For this review, take the finished solid that the model builds, in its own axes (mm). Face numbers are marked on the shaded views. A direction names the side the tool comes from. Round coordinates to 2 decimals unless told otherwise and drop trailing zeros. Write each loop counter-clockwise with the first axis right and the second up, starting at its lowest first coordinate (ties: lowest second). Pieces come first, ordered by that corner, then holes. Notation, with made-up numbers: (29, -37) -> (65, -37) arc R12 ccw to (65, -29) -> close; hole circle Ø9 at (14.5, 20). An arc over 180 degrees is marked (long way). Write each question's results on one line, items separated by ' | '. Start each with the question number.
Item 1: Add section C-C (y = -2). State the section outline as (x, z) points, plus the area to 3 significant figures.
Item 2: Add section D-D (x = 57). State the section outline as (y, z) points.
Item 3: Tool access review of the marked faces 1, 2, 3 and 4: name each direction out of +Z, -Z, +X, -X, +Y, -Y from which nothing blocks a thin tool from reaching the whole face with its end or side.
Item 4: Clearance check with flat-ended pins moving along their axes: pin 1 (3 mm diameter, centred on x = 115.5, y = 4.5, fed in from -Z); pin 2 (3 mm diameter, centred on x = 72, y = 13.5, fed in from +Z); pin 3 (12 mm diameter, centred on x = 4.5, z = -2, fed in from -Y); pin 4 (9 mm diameter, centred on x = 0, z = 0, fed in from +Y). State where each tip first meets the part, or that it passes through.
Item 5: Add section B-B (z = 0). State the section outline as (x, y) points, plus the area to 3 significant figures.
Item 6: Add section A-A (x = 0). State the section outline as (y, z) points, plus the area to 3 significant figures.
Item 7: To check wall thickness, follow line 1 along X through (y, z) = (7, -3); line 2 along X through (y, z) = (10, 11); line 3 along Z through (x, y) = (117.5, 16.5). State the ranges of each line that lie inside material, in increasing order.
from build123d import *

# Parameters (mm, degrees)
SKETCH2_W            = 178
SKETCH2_H            = 18
BOSS_EXTRUDE1_DEPTH  = 9
SWEEP2_PROFILE_R     = 12
SWEEP3_PROFILE_R     = 17.5
CUT_EXTRUDE1_DEPTH   = 6.5
CUT_SWEEP1_PROFILE_R = 7.5
CUT_SWEEP2_PROFILE_R = 12
FILLET1_R            = 24


with BuildPart() as part:
    # Sketch2 → Boss-Extrude1 (new body, symmetric)
    with BuildSketch(Plane.XY):
        with Locations((89, 9)):
            Rectangle(SKETCH2_W, SKETCH2_H)
    extrude(amount=BOSS_EXTRUDE1_DEPTH, both=True)

    # Sweep2: sweep along a path in Sketch11
    with BuildLine(Plane.XY) as sweep2_path:
        Line((0, -5), (0, 23))
    # Sweep2 profile (on start of the path) → Sweep2 (sweep)
    with BuildSketch(Plane(origin=(0, -5, 0), x_dir=(1, 0, 0), z_dir=(0, 1, 0))):
        Circle(SWEEP2_PROFILE_R)
    sweep(path=sweep2_path.line)

    # Sweep3: sweep along a path in Sketch18
    with BuildLine(Plane.XY) as sweep3_path:
        Line((178.00925882, 30), (178.00925882, -12))
    # Sweep3 profile (on start of the path) → Sweep3 (sweep)
    with BuildSketch(Plane(origin=(178.00925882, 30, 0), x_dir=(0, 0, -1), z_dir=(0, -1, 0))):
        Circle(SWEEP3_PROFILE_R)
    sweep(path=sweep3_path.line)

    # Sketch25 → Cut-Extrude1 (cut)
    with BuildSketch(Plane(origin=(0, 18, 0), x_dir=(1, 0, 0), z_dir=(0, 1, 0))):
        with BuildLine():
            Line((20.469090867, 5), (150.469090867, 5))
            ThreePointArc((150.469090867, 5), (155.469090867, 0), (150.469090867, -5))
            Line((150.469090867, -5), (20.469090867, -5))
            ThreePointArc((20.469090867, -5), (15.469090867, 0), (20.469090867, 5))
        make_face()
    cut_extrude1 = extrude(amount=-CUT_EXTRUDE1_DEPTH, mode=Mode.SUBTRACT)

    # Mirror1: Cut-Extrude1 across plane
    add(cut_extrude1.mirror(Plane.ZX.offset(9)), mode=Mode.SUBTRACT)

    # Cut-Sweep1: sweep along a path in Sketch11<2>
    with BuildLine(Plane.XY) as cut_sweep1_path:
        Line((0, -5), (0, 23))
    # Cut-Sweep1 profile (on start of the path) → Cut-Sweep1 (sweep, cut)
    with BuildSketch(Plane(origin=(0, -5, 0), x_dir=(1, 0, 0), z_dir=(0, 1, 0))):
        Circle(CUT_SWEEP1_PROFILE_R)
    sweep(path=cut_sweep1_path.line, mode=Mode.SUBTRACT)

    # Cut-Sweep2: sweep along a path in Sketch18<2>
    with BuildLine(Plane.XY) as cut_sweep2_path:
        Line((178.00925882, 30), (178.00925882, -12))
    # Cut-Sweep2 profile (on start of the path) → Cut-Sweep2 (sweep, cut)
    with BuildSketch(Plane(origin=(178.00925882, 30, 0), x_dir=(0, 0, -1), z_dir=(0, -1, 0))):
        Circle(CUT_SWEEP2_PROFILE_R)
    sweep(path=cut_sweep2_path.line, mode=Mode.SUBTRACT)

    # Fillet1
    fillet1_edges = [part.edges().sort_by_distance(p)[0] for p in [
        (7.937253933, 9, -9),
        (7.937253933, 9, 9),
        (163.0009278, 9, -9),
        (163.0009278, 9, 9),
    ]]
    fillet(fillet1_edges, radius=FILLET1_R)


solid = part.part
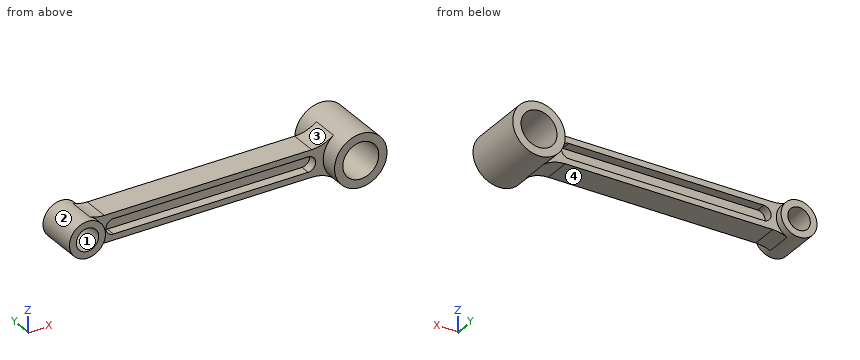
Responses:
1) outline: circle Ø24 at (0, 0); circle Ø35 at (178.01, 0); hole circle Ø15 at (0, 0); hole circle Ø24 at (178.01, 0) | area: 785 mm^2
2) outline: (0, -9) -> (18, -9) -> (18, -5) -> (11.5, -5) -> (11.5, 5) -> (18, 5) -> (18, 9) -> (0, 9) -> (0, 5) -> (6.5, 5) -> (6.5, -5) -> (0, -5) -> close
3) face 1: +Y, -Y | face 2: none | face 3: +Z, +Y, -Y | face 4: -Z, +Y, -Y
4) pin 1: stops at z = -9 | pin 2: stops at z = 9 | pin 3: stops at y = -5 | pin 4: passes through
5) outline: (-12, -5) -> (-7.5, -5) -> (-7.5, 23) -> (-12, 23) -> close; (7.5, -5) -> (12, -5) -> (12, 0) -> (15.47, 0) -> (15.47, 6.5) -> (155.47, 6.5) -> (155.47, 0) -> (160.51, 0) -> (160.51, -12) -> (166.01, -12) -> (166.01, 30) -> (160.51, 30) -> (160.51, 18) -> (155.47, 18) -> (155.47, 11.5) -> (15.47, 11.5) -> (15.47, 18) -> (12, 18) -> (12, 23) -> (7.5, 23) -> close; (190.01, -12) -> (195.51, -12) -> (195.51, 30) -> (190.01, 30) -> close | area: 1,570 mm^2
6) outline: (-5, -12) -> (23, -12) -> (23, -7.5) -> (-5, -7.5) -> close; (-5, 7.5) -> (23, 7.5) -> (23, 12) -> (-5, 12) -> close | area: 252 mm^2
7) line 1: x = -11.62 to -6.87, 6.87 to 166.39, 189.63 to 195.25 | line 2: x = -4.8 to 4.8, 162.44 to 173.21, 182.81 to 191.62 | line 3: z = -9 to -5, 5 to 9
